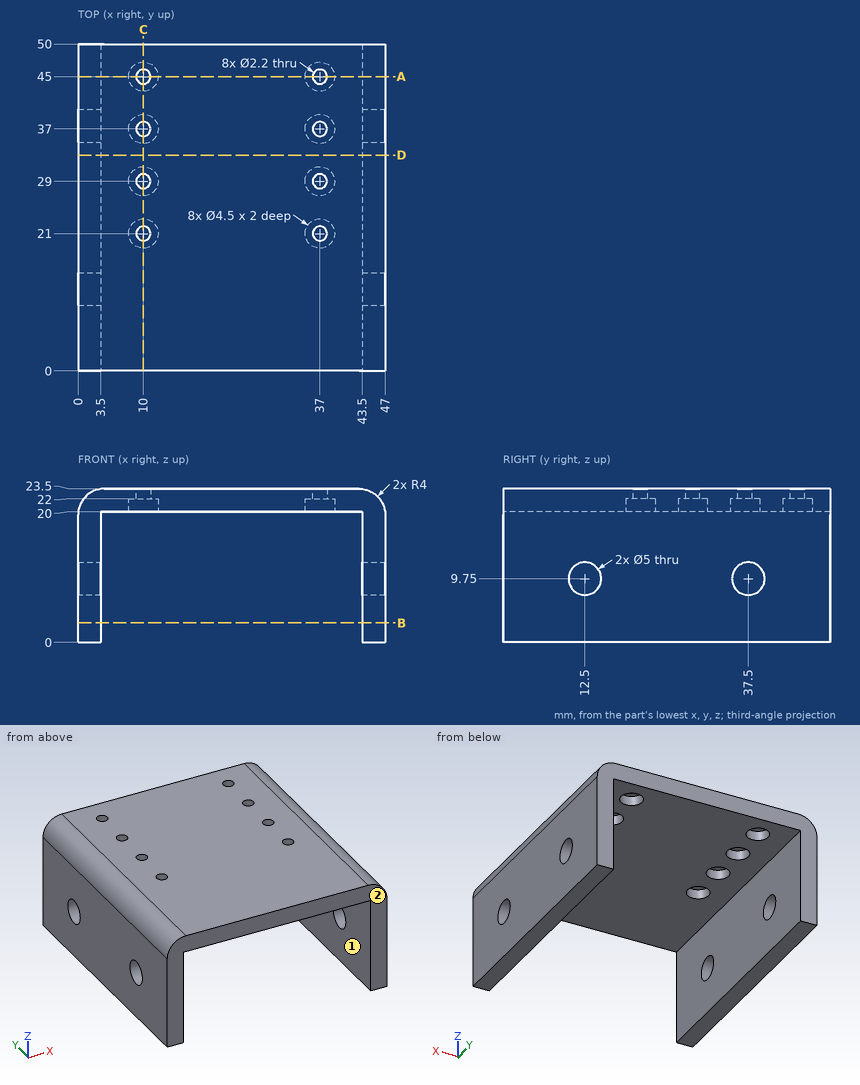
Verification items for this drawing (mm, ordinates from the low corner). A direction names the side the tool comes from. Give positions to 0.01 mm unless a question says otherwise; leave off trailing zeros. Write each loop counter-clockwise with the first axis right and the second up, starting at its lowest first coordinate (ties: lowest second). Pieces come first, ordered by that corner, then holes.
1) Section check C-C, the plane x = 10. State how many separate pieces and enclosed holes the cut face has, and give its area (3 significant figures).
2) Section check A-A, the plane y = 45. Record the boundary of the cut face in (x, z).
3) Access from +Z, -Z, +X, -X, +Y, -Y to the whole of each face (thin tool, end or side, straight path). Record for the marked faces 1 and 2.
4) Gauge pin test, flat ends, axial feed: pin 1 (2.5 mm diameter, centred on x = 10, y = 21, fed in from -Z); pin 2 (7 mm diameter, centred on x = 10, y = 29, fed in from -Z); pin 3 (2 mm diameter, centred on x = 10, y = 21, fed in from -Z). Record the tip position at first contact, or that the pin passes through.
5) Section check B-B, the plane z = 3. Record the boundary of the cut face in (x, y).
6) Section check D-D, the plane y = 33. Record the boundary of the cut face in (x, z), and give its area (3 significant figures).
7) Material ranges on L1, parallel to Y at x = 37, z = 23; L2, parallel to X at y = 31, z = 10; L3, parallel to Z at x = 40, y = 25, recorded low to high.
Computed:
1. separate pieces: 5
1. enclosed holes: 0
1. area: 126 mm2
2. outline: (0, 0) - (3.5, 0) - (3.5, 20) - (7.75, 20) - (7.75, 22) - (8.9, 22) - (8.9, 23.5) - (4, 23.5) arc R4 ccw to (0, 19.5) - close; (11.1, 22) - (12.25, 22) - (12.25, 20) - (34.75, 20) - (34.75, 22) - (35.9, 22) - (35.9, 23.5) - (11.1, 23.5) - close; (38.1, 22) - (39.25, 22) - (39.25, 20) - (43.5, 20) - (43.5, 0) - (47, 0) - (47, 19.5) arc R4 ccw to (43, 23.5) - (38.1, 23.5) - close
3. face 1: -Z, +Y, -Y
3. face 2: +Z, -Z, +X, -X, -Y
4. pin 1: stops at z = 22
4. pin 2: stops at z = 20
4. pin 3: passes through
5. outline: (0, 0) - (3.5, 0) - (3.5, 50) - (0, 50) - close; (43.5, 0) - (47, 0) - (47, 50) - (43.5, 50) - close
6. outline: (0, 0) - (3.5, 0) - (3.5, 20) - (43.5, 20) - (43.5, 0) - (47, 0) - (47, 19.5) arc R4 ccw to (43, 23.5) - (4, 23.5) arc R4 ccw to (0, 19.5) - close
6. area: 298 mm2
7. L1: y = 0 to 19.9, 22.1 to 27.9, 30.1 to 35.9, 38.1 to 43.9, 46.1 to 50
7. L2: x = 0 to 3.5, 43.5 to 47
7. L3: z = 20 to 23.5
